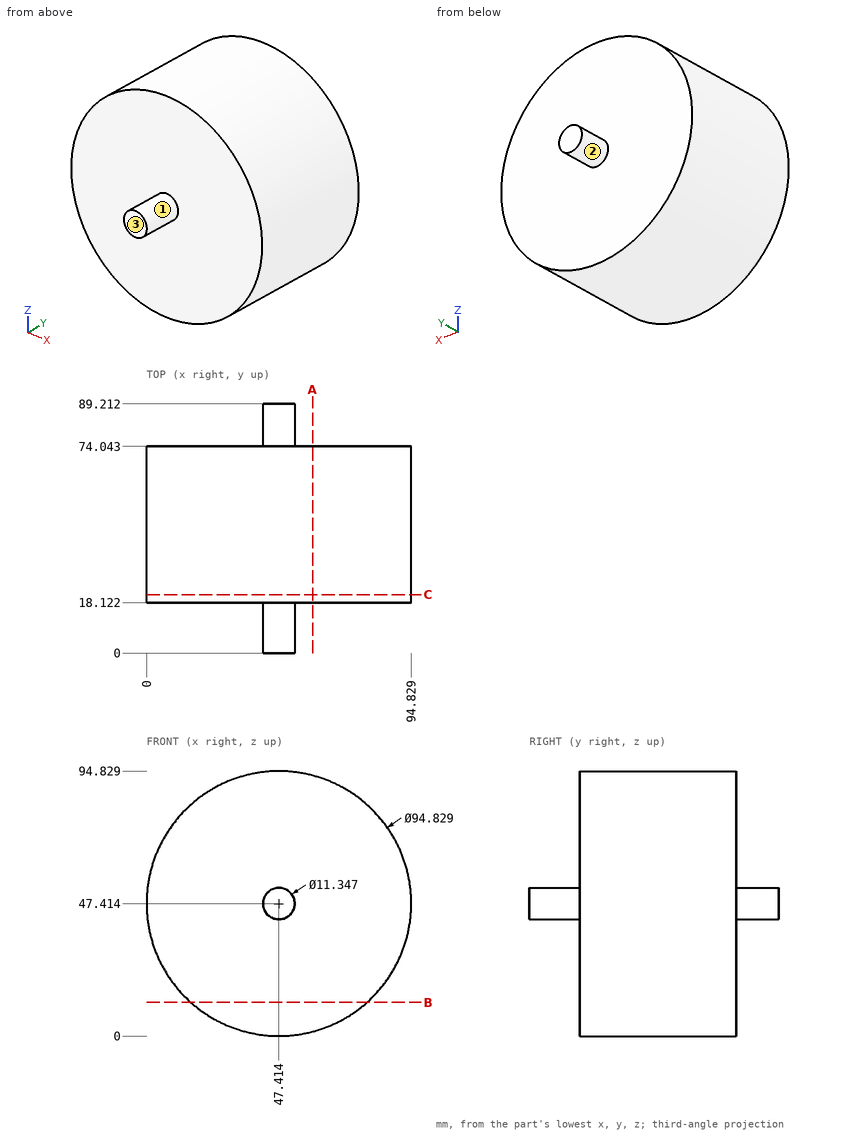
Design review of the part shown in the three views and the two pictorial views. Dimensions are in mm from the part's minimum x, y and z. A direction names the side the tool comes from. Round coordinates to 2 decimals unless told otherwise and drop trailing zeros. Order: outer loops, then holes, each group sorted by start corner. A loop starts at its lowest first (then second) coordinate and runs counter-clockwise, first axis right, second up. Notation, with made-up numbers: (-16.75, 13.25) - (35.25, 13.25) arc R13 ccw to (35.25, 17.25) - close; hole circle Ø1 at (15.25, -28.5). An arc over 180 degrees is marked (long way). One line per question, with ' | ' between items.
Item 1: For P1, Ø2, axis at x = 39, z = 68.5, coming from the +Y side; P2, Ø1, axis at y = 58, z = 22, coming from the +X side (1 decimal); P3, Ø1.5, axis at y = 65.5, z = 30, coming from the +X side; P4, Ø8, axis at x = 77, y = 79, coming from the +Z side, all flat-tipped, find the tip position at first contact; note any pin that passes through.
Checks:
P1: y = 74.04 | P2: x = 87.8 | P3: x = 91.8 | P4: through
Item 2: Take a section at C-C, the plane y = 21. Write out the cut boundary in (x, z) (1 decimal), then the cut area to 3 significant figures.
Checks:
outline: circle Ø94.8 at (47.4, 47.4) | area: 7,060 mm²
Item 3: Wall thickness on line 1 (Y direction, x = 44, z = 21.5); line 2 (Z direction, x = 44, y = 82) (1 decimal); line 3 (X direction, y = 58, z = 43) (1 decimal): over which ranges is each line inside the solid? List them lowest first. Write a range as [from, to].
Checks:
line 1: [18.12, 74.04] | line 2: [42.9, 51.9] | line 3: [0.2, 94.6]
Item 4: Take a section at B-B, the plane z = 12. Write out the cut boundary in (x, y), then the cut area to 3 significant figures.
Checks:
outline: (15.89, 18.12) - (78.94, 18.12) - (78.94, 74.04) - (15.89, 74.04) - close | area: 3,530 mm²
Item 5: Take a section at A-A, the plane x = 59.5. Write out the cut boundary in (y, z), then the cut area to 3 significant figures.
Checks:
outline: (18.12, 1.57) - (74.04, 1.57) - (74.04, 93.26) - (18.12, 93.26) - close | area: 5,130 mm²
Item 6: Machinability: for the marked faces 1, 2 and 3, which of the approach directions +Z, -Z, +X, -X, +Y, -Y give a long, thin tool a straight path to every point of the face, cutting with its end or side? Answer none if there is none.
Checks:
face 1: -Y | face 2: +Y | face 3: +Z, -Z, +X, -X, -Y
